from build123d import *

# Parameters (mm, degrees)
SKETCH_W        = 37.3
SKETCH_H        = 37.3
PAD_DEPTH       = 1
SKETCH001_R     = 1.15
POCKET_DEPTH    = 1.001
SKETCH002_W     = 24
SKETCH002_H     = 24
SKETCH002_W_2   = 22
SKETCH002_H_2   = 22
PAD001_DEPTH    = 1
POCKET001_DEPTH = 5
SKETCH004_W     = 9.5
SKETCH004_H     = 4
POCKET002_DEPTH = 5
SKETCH005_W     = 1.5
SKETCH005_H     = 2.5
PAD002_DEPTH    = 2
SKETCH006_W     = 12.5
SKETCH006_H     = 2.5
PAD003_DEPTH    = 1.5
PAD004_DEPTH    = 19
SKETCH008_W     = 18.5
SKETCH008_H     = 3
PAD006_DEPTH    = 1.5
SKETCH009_W     = 22
SKETCH009_H     = 6
PAD007_DEPTH    = 2
SKETCH010_W     = 6
SKETCH010_H     = 1
PAD008_DEPTH    = 27
SKETCH011_W     = 6
SKETCH011_H     = 1
PAD009_DEPTH    = 4.5
SKETCH012_W     = 6
SKETCH012_H     = 7
PAD010_DEPTH    = 1
SKETCH013_W     = 7
SKETCH013_H     = 7
PAD011_DEPTH    = 1
SKETCH014_W     = 7
SKETCH014_H     = 7
PAD012_DEPTH    = 1


with BuildPart() as part:
    # Sketch → Pad (new body)
    with BuildSketch(Plane.XY):
        Rectangle(SKETCH_W, SKETCH_H)
    extrude(amount=PAD_DEPTH)

    # Sketch001 (on Face6 of Pad) → Pocket (cut, through all)
    with BuildSketch(Plane.XY.offset(1)):
        with Locations((15.8, 15.8)):
            Circle(SKETCH001_R)
        with Locations((-15.8, -15.8)):
            Circle(SKETCH001_R)
        with Locations((15.8, -15.8)):
            Circle(SKETCH001_R)
        with Locations((-15.8, 15.8)):
            Circle(SKETCH001_R)
    extrude(amount=-POCKET_DEPTH, mode=Mode.SUBTRACT)

    # Sketch002 (on Face5 of Pocket) → Pad001 (join)
    with BuildSketch(Plane.XY.offset(1)):
        Rectangle(SKETCH002_W, SKETCH002_H)
        Rectangle(SKETCH002_W_2, SKETCH002_H_2, mode=Mode.SUBTRACT)
    extrude(amount=PAD001_DEPTH)

    # Sketch003 (on Face20 of Pad001) → Pocket001 (cut)
    with BuildSketch(Plane.XY.offset(1)):
        Polygon((-11, -3), (-11, -8), (11, -8), (11, -3), (5, -3), (5, -2), (9.25, -2), (9.25, 5), (-9.25, 5), (-9.25, -2), (-5, -2), (-5, -3), align=None)
    extrude(amount=-POCKET001_DEPTH, mode=Mode.SUBTRACT)

    # Sketch004 (on Face25 of Pocket001) → Pocket002 (cut)
    with BuildSketch(Plane.XY.offset(1)):
        with Locations((0, 8)):
            Rectangle(SKETCH004_W, SKETCH004_H)
    extrude(amount=-POCKET002_DEPTH, mode=Mode.SUBTRACT)

    # Sketch005 (on Face31 of Pocket002) → Pad002 (join)
    with BuildSketch(Plane.XY.offset(1)):
        with Locations((-5.5, 8)):
            Rectangle(SKETCH005_W, SKETCH005_H)
        with Locations((5.5, 8)):
            Rectangle(SKETCH005_W, SKETCH005_H)
    extrude(amount=PAD002_DEPTH)

    # Sketch006 (on Face40 of Pad002) → Pad003 (join)
    with BuildSketch(Plane.XY.offset(3)):
        with Locations((0, 8)):
            Rectangle(SKETCH006_W, SKETCH006_H)
    extrude(amount=PAD003_DEPTH)

    # Sketch007 (on Face31 of Pad003) → Pad004 (join)
    with BuildSketch(Plane.XY.offset(1)):
        Polygon((-11, 3), (-11, -3), (-5, -3), (-5, -2), (-9.25, -2), (-9.25, 3), align=None)
        Polygon((9.25, 3), (9.25, -2), (5, -2), (5, -3), (11, -3), (11, 3), align=None)
    extrude(amount=PAD004_DEPTH)

    # Sketch008 (on Face31 of Pad004) → Pad006 (join)
    with BuildSketch(Plane.XY.offset(20)):
        Polygon((-11, 3), (-11, 2), (-11, -1), (-11, -3), (11, -3), (11, 3), align=None)
        with Locations((0, 0.5)):
            Rectangle(SKETCH008_W, SKETCH008_H, mode=Mode.SUBTRACT)
    extrude(amount=PAD006_DEPTH)

    # Sketch009 → Pad007 (join)
    with BuildSketch(Plane.XY.offset(21.5)):
        Rectangle(SKETCH009_W, SKETCH009_H)
    extrude(amount=PAD007_DEPTH)

    # Sketch010 (on Face42 of Pad007) → Pad008 (join)
    with BuildSketch(Plane.XY.offset(1)):
        with Locations((-8, -8.5)):
            Rectangle(SKETCH010_W, SKETCH010_H)
        with Locations((8, -8.5)):
            Rectangle(SKETCH010_W, SKETCH010_H)
    extrude(amount=PAD008_DEPTH)

    # Sketch011 (on Face19 of Pad008) → Pad009 (join)
    with BuildSketch(Plane.XY.offset(23.5)):
        with Locations((-8, -2.5)):
            Rectangle(SKETCH011_W, SKETCH011_H)
        with Locations((8, -2.5)):
            Rectangle(SKETCH011_W, SKETCH011_H)
    extrude(amount=PAD009_DEPTH)

    # Sketch012 (on Face62 of Pad009) → Pad010 (join)
    with BuildSketch(Plane.XY.offset(28)):
        with Locations((-8, -5.5)):
            Rectangle(SKETCH012_W, SKETCH012_H)
        with Locations((8, -5.5)):
            Rectangle(SKETCH012_W, SKETCH012_H)
    extrude(amount=PAD010_DEPTH)

    # Sketch013 (on Face54 of Pad010) → Pad011 (join)
    with BuildSketch(Plane(origin=(-11, 0, 0), x_dir=(0, -1, 0), z_dir=(-1, 0, 0))):
        with Locations((5.5, 15.5)):
            Rectangle(SKETCH013_W, SKETCH013_H)
    extrude(amount=PAD011_DEPTH)

    # Sketch014 (on Face18 of Pad011) → Pad012 (join)
    with BuildSketch(Plane.YZ.offset(11)):
        with Locations((-5.5, 15.5)):
            Rectangle(SKETCH014_W, SKETCH014_H)
    extrude(amount=PAD012_DEPTH)


solid = part.part
Here's how the part is built. I have some questions about the finished solid (model axes, mm). A direction names the side the tool comes from. Round coordinates to 2 decimals unless told otherwise and drop trailing zeros. Loops run counter-clockwise (first coordinate to the right, second up) from the corner with the lowest first, then second, coordinate; pieces in that order, holes last.
1. If I drill on line 1 along Y through (x, z) = (15.8, 0.55); line 2 along Y through (x, z) = (-6.5, 8.5); line 3 along Z through (x, y) = (-14.5, 16.5), over which ranges is the centre line in solid material (lowest first)?
Answer list:
line 1: y = -18.65 to -16.95, -14.65 to 14.65, 16.95 to 18.65
line 2: y = -9 to -8, -3 to -2
line 3: z = 0 to 1
2. If we section it at D-D on x = 3: Count the separate pieces of the cut face and the enclosed holes in it, plus the area to 4 significant figures.
Answer list:
separate pieces: 5
enclosed holes: 0
area: 42.55 mm2
3. If we section it at C-C on z = 7.75: Write out the boundary of the cut face in (x, y), plus the area to 3 significant figures.
Answer list:
outline: (-11, -9) - (-5, -9) - (-5, -8) - (-11, -8) - close; (-11, -3) - (-5, -3) - (-5, -2) - (-9.25, -2) - (-9.25, 3) - (-11, 3) - close; (5, -9) - (11, -9) - (11, -8) - (5, -8) - close; (5, -3) - (11, -3) - (11, 3) - (9.25, 3) - (9.25, -2) - (5, -2) - close
area: 41.5 mm2
4. For P1, Ø1.8, axis at x = -15.8, y = 15.8, coming from the -Z side; P2, Ø6, axis at x = 9.5, z = 25, coming from the +Y side; P3, Ø5, axis at y = -9.5, z = 25, coming from the -X side; P4, Ø3.5, axis at y = -7, z = 15, coming from the +X side, each with a flat end and sliding along its axis, tell me the tip position at first contact or that it passes through.
Answer list:
P1: passes through
P2: stops at y = 3
P3: stops at x = -11
P4: stops at x = 12
5. Which directions (+Z, -Z, +X, -X, +Y, -Y) give clear straight access to the entire face, cutting with the end or side of a thin tool? Please do faces 1 (the face through (-0.2, 11, 1.5)), 2 (the face through (0, 8, 3)), 3 (the face through (-12, -5, 16)).
Answer list:
face 1: +Z
face 2: -Z, +Y, -Y
face 3: +Z, -X, +Y, -Y
6. We'd pull the mould along X, two halves only. Please class faces 4 (the face through (11, -10, 1.5)), 5 (the face through (-8, -5, 28)), 6 (the face through (-12, -0.2, 1.5)): +X half, -X half, draft (parallel to the pull), parting line (faces both ways), or undercut.
Answer list:
face 4: undercut
face 5: draft
face 6: -X half
7. If we section it at A-A on y = -15.8: Write out the boundary of the cut face in (x, z).
Answer list:
outline: (-18.65, 0) - (-16.95, 0) - (-16.95, 1) - (-18.65, 1) - close; (-14.65, 0) - (14.65, 0) - (14.65, 1) - (-14.65, 1) - close; (16.95, 0) - (18.65, 0) - (18.65, 1) - (16.95, 1) - close
